```python
from build123d import *

# Parameters (mm, degrees)
F0_W     = 75
F0_H     = 125
F1_DEPTH = 625
F2_R     = 17.5
F3_DEPTH = 1250
F4_R     = 25


with BuildPart() as f1:
    # F0 (on Front) → F1 (new body, symmetric)
    with BuildSketch(Plane.XZ):
        Rectangle(F0_W, F0_H)
    extrude(amount=F1_DEPTH, both=True)

    # F2 (on face) → F3 (cut)
    with BuildSketch(Plane.XZ.offset(625)):
        Circle(F2_R)
    extrude(amount=-F3_DEPTH, mode=Mode.SUBTRACT)

    # F4
    f4_edges = [f1.edges().sort_by_distance(p)[0] for p in [
        (37.5, 0, 62.5),
        (-37.5, 0, 62.5),
        (-37.5, 0, -62.5),
        (37.5, 0, -62.5),
    ]]
    fillet(f4_edges, radius=F4_R)


solid = f1.part
```
Source: CAD feature listing. Evaluate the final solid. Frame: model axes, mm. Give positions to 0.01 mm unless a question says otherwise; leave off trailing zeros. Write each loop counter-clockwise with the first axis right and the second up, starting at its lowest first coordinate (ties: lowest second). Pieces come first, ordered by that corner, then holes.
1. Pull-direction query (Z, two-part tool) for faces 1 (the face through (29.982, 8.75, 55.371)), 2 (the face through (-30.371, -8.75, -54.982)), 3 (the face through (-13.887, -8.75, -10.648)); classes: +Z half, -Z half, draft (parallel to the pull), parting line (faces both ways), or undercut.
2. Material intervals for line 1 along Z through (x, y) = (2.5, 386.5); line 2 along Z through (x, y) = (0, 250); line 3 along X through (y, z) = (212, -13.5), sorted ascending.
3. Section query C-C (y = -374). Return the cut outline in (x, z).
4. Section query A-A (x = 0). Return the cut outline in (y, z), then the cut area to 4 significant figures.
5. Section query B-B (z = 0). Return the cut outline in (x, y), then the cut area to 3 significant figures.
6. First-contact query: pin 1 (3 mm diameter, centred on x = -28, y = 131, fed in from -Z); pin 2 (10 mm diameter, centred on x = -29.5, y = -163.5, fed in from -Z). Flat tips, straight axial feed; report the tip coordinate or a pass-through.
7. Section query D-D (z = 49.5). Return the cut outline in (x, y), then the cut area to 3 significant figures.
Output values:
1. face 1: +Z half
1. face 2: -Z half
1. face 3: undercut
2. line 1: z = -62.5 to -17.32, 17.32 to 62.5
2. line 2: z = -62.5 to -17.5, 17.5 to 62.5
2. line 3: x = -37.5 to -11.14, 11.14 to 37.5
3. outline: (-37.5, -37.5) arc R25 ccw to (-12.5, -62.5) - (12.5, -62.5) arc R25 ccw to (37.5, -37.5) - (37.5, 37.5) arc R25 ccw to (12.5, 62.5) - (-12.5, 62.5) arc R25 ccw to (-37.5, 37.5) - close; hole circle Ø35 at (0, 0)
4. outline: (-625, -62.5) - (625, -62.5) - (625, -17.5) - (-625, -17.5) - close; (-625, 17.5) - (625, 17.5) - (625, 62.5) - (-625, 62.5) - close
4. area: 112,500 mm2
5. outline: (-37.5, -625) - (-17.5, -625) - (-17.5, 625) - (-37.5, 625) - close; (17.5, -625) - (37.5, -625) - (37.5, 625) - (17.5, 625) - close
5. area: 50,000 mm2
6. pin 1: stops at z = -58.21
6. pin 2: stops at z = -59.43
7. outline: (-34.43, -625) - (34.43, -625) - (34.43, 625) - (-34.43, 625) - close
7. area: 86,100 mm2
